from build123d import *

# Parameters (mm, degrees)
F1_DEPTH = 9
F2_W     = 0.1
F2_H     = 4.4654227124
F4_R     = 0.75
F5_DEPTH = 2.501


with BuildPart() as f1:
    # F0 (on Front) → F1 (new body)
    with BuildSketch(Plane.XZ):
        Polygon((-1.25, 12), (-1.25, 0), (1.25, 0), (1.25, 8.3), align=None)
    extrude(amount=F1_DEPTH)

    # F2 (on face) → F3 (revolve, cut)
    with BuildSketch(Plane(origin=(4.7085005015, 0, 3.1814192578), x_dir=(0, 1, 0), z_dir=(0.8285889687, 0, 0.5598574113))):
        with Locations((-4.55, 8.4101780322)):
            Rectangle(F2_W, F2_H)
    revolve(axis=Axis((0, -4.5, 10.15), (0.5598574113, 0, -0.8285889687)), mode=Mode.SUBTRACT)

    # F4 (on face) → F5 (cut, through all)
    with BuildSketch(Plane.YZ.offset(1.25)):
        with Locations((-4.6, 4.15)):
            Circle(F4_R)
    extrude(amount=-F5_DEPTH, mode=Mode.SUBTRACT)


solid = f1.part
Source: CAD feature listing. Evaluate the final solid. Frame: model axes, mm. Round coordinates to 2 decimals unless told otherwise and drop trailing zeros. Loops run counter-clockwise (first coordinate to the right, second up) from the corner with the lowest first, then second, coordinate; pieces in that order, holes last. Notation, with made-up numbers: M -13,57 L 23,57 A20 ccw 23,73 Z; hole C 21.25,43.25 d5. An arc over 180 degrees is marked long. Return JSON: item names as keys, results as strings. Group by question number.
1. Material intervals for line 1 along Y through (x, z) = (-0.45, 10.75); line 2 along Z through (x, y) = (0.85, -4); line 3 along Z through (x, y) = (0.8, -4), sorted ascending. Write a range as from..to.
2. Section query A-A on z = 4.15. Output: boundary loops of the cut face in (x, y), and give its area (4 significant figures).
3. Section query B-B on y = -7.25. Output: boundary loops of the cut face in (x, z), and give its area (3 significant figures).
4. Mould query, pull axis Y, two halves, no side actions, for faces 1 (the face through (0.02, -3.91, 3.86)), 2 (the face through (0, -4, 0)), 3 (the face through (0, -9, 5)). Classes: released by +Y, released by -Y, zero draft, split by the parting line, or undercut.
Checks:
{
 "1": {"line 1": "y = -9..-4.59, -4.41..0", "line 2": "z = 0..3.7, 4.6..8.89", "line 3": "z = 0..3.7, 4.6..8.97"},
 "2": {"outline": "M -1.25,-9 L 1.25,-9 L 1.25,-5.35 L -1.25,-5.35 Z; M -1.25,-3.85 L 1.25,-3.85 L 1.25,0 L -1.25,0 Z", "area": "18.75 mm²"},
 "3": {"outline": "M -1.25,0 L 1.25,0 L 1.25,8.3 L -1.25,12 Z", "area": "25.4 mm²"},
 "4": {"face 1": "undercut", "face 2": "zero draft", "face 3": "released by -Y"}
}
